Check sheet for the modelled part. Datum: model origin and axes. Units: mm. A direction names the side the tool comes from. Give positions to 0.01 mm unless a question says otherwise; leave off trailing zeros. Write each loop counter-clockwise with the first axis right and the second up, starting at its lowest first coordinate (ties: lowest second). Pieces come first, ordered by that corner, then holes. Notation, with made-up numbers: (87, -18.5) -> (100, -18.5) arc R20 ccw to (100, -14.5) -> close; hole circle Ø5 at (20.5, 6.25). An arc over 180 degrees is marked (long way). Use a Markdown table: item, result. Add a question column.
1. Release check for a two-part mould opening along Y. For faces 1 (the flat face through (0, 50, 5)), 2 (the flat face through (0, -32, 10)), 3 (the flat face through (0, -11.5, 15)) record: released by +Y, released by -Y, zero draft, split by the parting line, or undercut.
2. Gauge pin test, flat ends, axial feed: P1, Ø2, axis at x = -0.5, y = -28.5, coming from the +Z side; P2, Ø4.5, axis at y = -4.5, z = 19.5, coming from the +X side; P3, Ø1.5, axis at y = 37, z = 6.5, coming from the -X side; P4, Ø10, axis at x = -2.5, z = 10.5, coming from the +Y side. Record the tip position at first contact, or that the pin passes through.
3. Scan lines: probe 1 along X at (y, z) = (-5.5, 12.25); probe 2 along Y at (x, z) = (16, 17); probe 3 along Y at (x, z) = (13, 7.5). Record each from-to range of solid material in increasing order. Write a range as [from, to].
4. Cross-section at A-A (z = 8.75). Enter the section's corners in (x, y).
5. Cross-section at C-C (y = 1.5). Enter the section's corners in (x, z), then the cut area to 4 significant figures.
6. Cross-section at D-D (z = 15). Enter the section's corners in (x, y).
7. Cross-section at B-B (x = 6). Enter the section's corners in (y, z).
8. Set-up check for faces 4 (the flat face through (-15, -32, 5)), 5 (the flat face through (-15, 33, 5)), 6 (the flat face through (32.5, 0, 17)), 7 (the flat face through (0, 0, 5)): record each of +Z, -Z, +X, -X, +Y, -Y from which the full face is reachable in a straight line by a thin tool's end or side.
from build123d import *

# Parameters (mm, degrees)
F1_DEPTH = 10
F3_DEPTH = 15
F4_W     = 35
F4_H     = 23
F5_DEPTH = 20


with BuildPart() as f1:
    # F0 (on Top) → F1 (new body)
    with BuildSketch(Plane.XY):
        Polygon((15, 15), (15, 50), (-15, 50), (-15, 15), (-50, 15), (-50, -15), (-15, -15), (-15, -50), (15, -50), (15, -15), (50, -15), (50, 15), align=None)
    extrude(amount=F1_DEPTH)

    # F2 (on face) → F3 (join)
    with BuildSketch(Plane.XY.offset(10)):
        Polygon((32.5, 15), (15, 15), (-15, 15), (-32.5, 15), (-32.5, -15), (-15, -15), (15, -15), (32.5, -15), align=None)
    extrude(amount=F3_DEPTH)

    # F4 (on face) → F5 (cut)
    with BuildSketch(Plane.XY.offset(25)):
        Rectangle(F4_W, F4_H)
    extrude(amount=-F5_DEPTH, mode=Mode.SUBTRACT)


solid = f1.part
Worked answers:
| question | item | result |
|---|---|---|
| 1 | face 1 | released by +Y |
| 1 | face 2 | zero draft |
| 1 | face 3 | undercut |
| 2 | P1 | stops at z = 10 |
| 2 | P2 | stops at x = 32.5 |
| 2 | P3 | stops at x = -15 |
| 2 | P4 | stops at y = 50 |
| 3 | probe 1 | x = [-32.5, -17.5], [17.5, 32.5] |
| 3 | probe 2 | y = [-15, -11.5], [11.5, 15] |
| 3 | probe 3 | y = [-50, -11.5], [11.5, 50] |
| 4 | outline | (-50, -15) -> (-15, -15) -> (-15, -50) -> (15, -50) -> (15, -15) -> (50, -15) -> (50, 15) -> (15, 15) -> (15, 50) -> (-15, 50) -> (-15, 15) -> (-50, 15) -> close; hole (-17.5, -11.5) -> (17.5, -11.5) -> (17.5, 11.5) -> (-17.5, 11.5) -> close |
| 5 | outline | (-50, 0) -> (50, 0) -> (50, 10) -> (32.5, 10) -> (32.5, 25) -> (17.5, 25) -> (17.5, 5) -> (-17.5, 5) -> (-17.5, 25) -> (-32.5, 25) -> (-32.5, 10) -> (-50, 10) -> close |
| 5 | area | 1,275 mm² |
| 6 | outline | (-32.5, -15) -> (32.5, -15) -> (32.5, 15) -> (-32.5, 15) -> close; hole (-17.5, -11.5) -> (17.5, -11.5) -> (17.5, 11.5) -> (-17.5, 11.5) -> close |
| 7 | outline | (-50, 0) -> (50, 0) -> (50, 10) -> (15, 10) -> (15, 25) -> (11.5, 25) -> (11.5, 5) -> (-11.5, 5) -> (-11.5, 25) -> (-15, 25) -> (-15, 10) -> (-50, 10) -> close |
| 8 | face 4 | +Z, -Z, -X, -Y |
| 8 | face 5 | +Z, -Z, -X, +Y |
| 8 | face 6 | +Z, +X, +Y, -Y |
| 8 | face 7 | +Z |
